The listing builds one solid part. Answer for the finished solid, in the listing's coordinates (mm). Face numbers are marked on the shaded views. A direction names the side the tool comes from. Coordinates: 2 decimals unless noted, no trailing zeros. Loops run counter-clockwise (first coordinate to the right, second up) from the corner with the lowest first, then second, coordinate; pieces in that order, holes last. Notation, with made-up numbers: (69.25, 21) - (119.25, 21) arc R16 cw to (119.25, 52) - close; hole circle Ø1 at (72, 10.5). An arc over 180 degrees is marked (long way). Return JSON: item names as keys, results as strings. Group by question number.
1. Find the intervals of material crossed by line 1 along Y through (x, z) = (-5.25, 33.5); line 2 along X through (y, z) = (0, 1.2) (3 decimals); line 3 along Y through (x, z) = (0, 0.85), in increasing order.
2. Section B-B (x = -7.5) is taken. Write down the section's boundary in (y, z).
3. Section C-C (x = 0) is taken. Write down the section's boundary in (y, z), and give its area (3 significant figures).
4. Section A-A (z = 33) is taken. Write down the section's boundary in (x, y) (3 decimals), and give its area (3 significant figures).
5. Which of the six approach directions +Z, -Z, +X, -X, +Y, -Y give full straight-line access (tool end or side, diameter ignored) to the marked faces 5 and 6?
6. The mould has two halves that part along X. Classify the marked faces 1, 2, 3 and 4: pulls with the +X half, pulls with the -X half, needs draft (parallel to the pull), parting line crosses it, or undercut.
7. Section D-D (y = -3.25) is taken. Write down the section's boundary in (x, z).
8. Each of these flat-tipped pins is pushed along its axis until it touches: P1, Ø0.8, axis at y = -3.5, z = 14, coming from the -X side; P2, Ø0.8, axis at y = -3.5, z = 17.5, coming from the +X side; P3, Ø6.5, axis at x = 1.5, z = 22.5, coming from the -Y side. Where does it stop, or does it pass through?
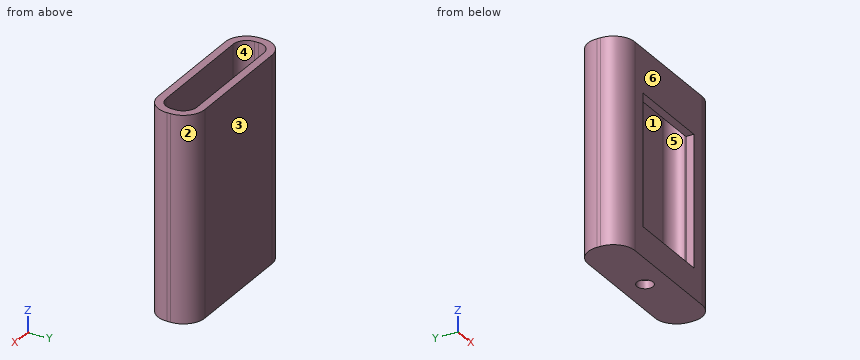
```python
from build123d import *

# Parameters (mm, degrees)
F1_DEPTH = 38
F2_T     = -1.5
F3_R     = 1.5
F4_DEPTH = 25
F5_W     = 16.002862
F5_H     = 24.337668
F6_DEPTH = 3


with BuildPart() as f1:
    # F0 (on Top) → F1 (new body)
    with BuildSketch(Plane.XY):
        with BuildLine():
            ThreePointArc((14.575, 0.36), (13.403427, 3.188427), (10.575, 4.36))
            Line((10.575, 4.36), (-10.575, 4.36))
            ThreePointArc((-10.575, 4.36), (-13.403427, 3.188427), (-14.575, 0.36))
            Line((-14.575, 0.36), (-14.575, -0.36))
            ThreePointArc((-14.575, -0.36), (-13.403427, -3.188427), (-10.575, -4.36))
            Line((-10.575, -4.36), (10.575, -4.36))
            ThreePointArc((10.575, -4.36), (13.403427, -3.188427), (14.575, -0.36))
            Line((14.575, -0.36), (14.575, 0.36))
        make_face()
    extrude(amount=F1_DEPTH)

    # F2
    f2_openings = [f1.faces().sort_by_distance(p)[0] for p in [
        (0, 0, 38),
    ]]
    offset(amount=F2_T, openings=f2_openings)

    # F3 (on Top) → F4 (cut)
    with BuildSketch(Plane.XY):
        Circle(F3_R)
    extrude(amount=F4_DEPTH, mode=Mode.SUBTRACT)

    # F5 (on face) → F6 (cut)
    with BuildSketch(Plane.XZ.offset(4.36)):
        with Locations((0, 17.704612)):
            Rectangle(F5_W, F5_H)
    extrude(amount=-F6_DEPTH, mode=Mode.SUBTRACT)


solid = f1.part
```
The answers:
{
 "1": {"line 1": "y = -4.36 to -2.86, 2.86 to 4.36", "line 2": "x = -14.575 to -1.5, 1.5 to 14.575", "line 3": "y = -4.36 to -1.5, 1.5 to 4.36"},
 "2": {"outline": "(-4.36, 0) - (4.36, 0) - (4.36, 38) - (2.86, 38) - (2.86, 1.5) - (-2.86, 1.5) - (-2.86, 5.54) - (-4.36, 5.54) - close; (-4.36, 29.87) - (-2.86, 29.87) - (-2.86, 38) - (-4.36, 38) - close"},
 "3": {"outline": "(-4.36, 0) - (-1.5, 0) - (-1.5, 1.5) - (-2.86, 1.5) - (-2.86, 5.54) - (-4.36, 5.54) - close; (-4.36, 29.87) - (-2.86, 29.87) - (-2.86, 38) - (-4.36, 38) - close; (1.5, 0) - (4.36, 0) - (4.36, 38) - (2.86, 38) - (2.86, 1.5) - (1.5, 1.5) - close", "area": "81.6 mm2"},
 "4": {"outline": "(-14.575, -0.36) arc R4 ccw to (-10.575, -4.36) - (10.575, -4.36) arc R4 ccw to (14.575, -0.36) - (14.575, 0.36) arc R4 ccw to (10.575, 4.36) - (-10.575, 4.36) arc R4 ccw to (-14.575, 0.36) - close; hole (-13.075, -0.36) arc R2.5 ccw to (-10.575, -2.86) - (10.575, -2.86) arc R2.5 ccw to (13.075, -0.36) - (13.075, 0.36) arc R2.5 ccw to (10.575, 2.86) - (-10.575, 2.86) arc R2.5 ccw to (-13.075, 0.36) - close", "area": "96.2 mm2"},
 "5": {"face 5": "+Z", "face 6": "+Z, -Z, +X, -X, -Y"},
 "6": {"face 1": "undercut", "face 2": "pulls with the +X half", "face 3": "needs draft", "face 4": "undercut"},
 "7": {"outline": "(-13.34, 0) - (13.34, 0) - (13.34, 38) - (-13.34, 38) - close; hole (-8, 5.54) - (8, 5.54) - (8, 29.87) - (-8, 29.87) - close"},
 "8": {"P1": "stops at x = -13.49", "P2": "stops at x = 13.49", "P3": "stops at y = 2.86"}
}
